Can you work these out from the drawing? Everything is in mm from the part's minimum corner. A direction names the side the tool comes from. Give positions to 0.01 mm unless a question says otherwise; leave off trailing zeros. Write each loop counter-clockwise with the first axis right and the second up, starting at its lowest first coordinate (ties: lowest second). Pieces come first, ordered by that corner, then holes. Notation, with made-up numbers: (25, 63) -> (69, 63) arc R20 ccw to (69, 81) -> close; hole circle Ø5 at (53, 23.25). An arc over 180 degrees is marked (long way). Return JSON: item names as keys, results as strings.
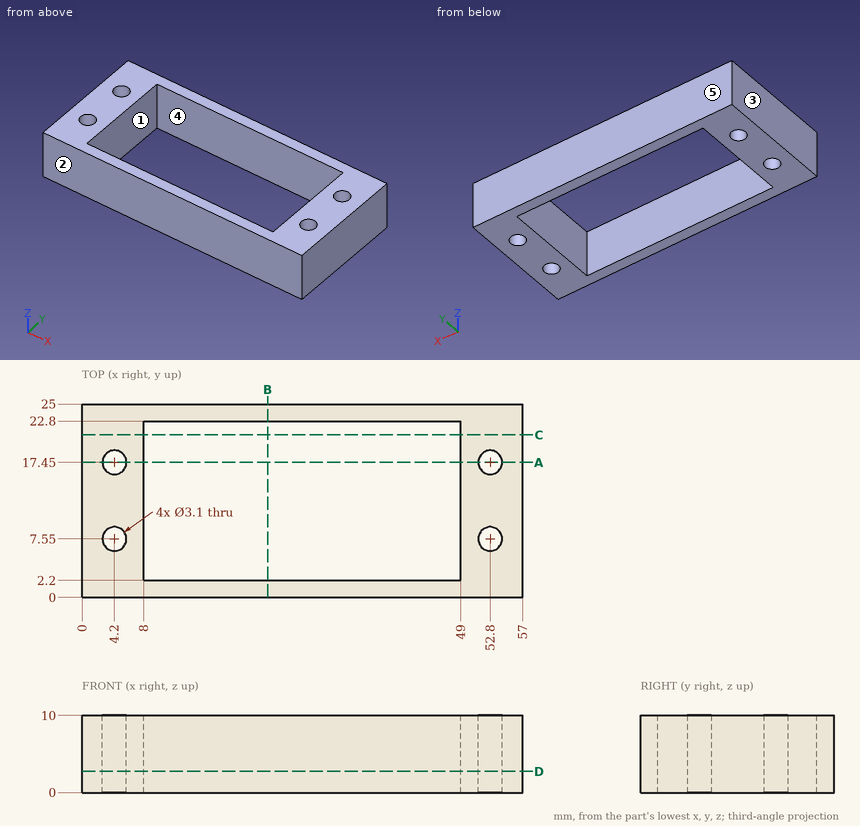
1. Suppose I cut it at B-B, the plane x = 24. List the corners of the cut face in (y, z) for me.
Taken from the geometry:
{"outline": "(0, 0) -> (2.2, 0) -> (2.2, 10) -> (0, 10) -> close; (22.8, 0) -> (25, 0) -> (25, 10) -> (22.8, 10) -> close"}
2. Which directions (+Z, -Z, +X, -X, +Y, -Y) give clear straight access to the entire face, cutting with the end or side of a thin tool? Please do the marked faces 4 and 5.
Taken from the geometry:
{"face 4": "+Z, -Z", "face 5": "+Z, -Z, +X, -X, +Y"}
3. If I drill on line 1 (Y direction, x = 4.2, z = 3); line 2 (X direction, y = 5.25, z = 1); line 3 (Y direction, x = 3, z = 5.25), over which ranges is the centre line in solid material (lowest first)? Write a range as [from, to].
Taken from the geometry:
{"line 1": "y = [0, 6], [9.1, 15.9], [19, 25]", "line 2": "x = [0, 8], [49, 57]", "line 3": "y = [0, 6.57], [8.53, 16.47], [18.43, 25]"}
4. Suppose I cut it at D-D, the plane z = 2.75. List the corners of the cut face in (x, y) for me.
Taken from the geometry:
{"outline": "(0, 0) -> (57, 0) -> (57, 25) -> (0, 25) -> close; hole circle Ø3.1 at (4.2, 7.55); hole circle Ø3.1 at (4.2, 17.45); hole (8, 2.2) -> (49, 2.2) -> (49, 22.8) -> (8, 22.8) -> close; hole circle Ø3.1 at (52.8, 7.55); hole circle Ø3.1 at (52.8, 17.45)"}
5. Suppose I cut it at A-A, the plane y = 17.45. List the corners of the cut face in (x, z) for me.
Taken from the geometry:
{"outline": "(0, 0) -> (2.65, 0) -> (2.65, 10) -> (0, 10) -> close; (5.75, 0) -> (8, 0) -> (8, 10) -> (5.75, 10) -> close; (49, 0) -> (51.25, 0) -> (51.25, 10) -> (49, 10) -> close; (54.35, 0) -> (57, 0) -> (57, 10) -> (54.35, 10) -> close"}
6. For pin 1 Ø1.9 at (x, y) = (52.8, 17.45) entering from -Z, with a flat end and sliding along its axis, tell me the tip position at first contact or that it passes through.
Taken from the geometry:
{"pin 1": "passes through"}
7. Suppose I cut it at C-C, the plane y = 21. List the corners of the cut face in (x, z) for me.
Taken from the geometry:
{"outline": "(0, 0) -> (8, 0) -> (8, 10) -> (0, 10) -> close; (49, 0) -> (57, 0) -> (57, 10) -> (49, 10) -> close"}
8. If we mould it in two halves opening along Y, with no side actions, what happens to the marked faces 1, 2 and 3? For each: released by +Y, released by -Y, zero draft, split by the parting line, or undercut.
Taken from the geometry:
{"face 1": "undercut", "face 2": "released by -Y", "face 3": "zero draft"}
